Check sheet for the modelled part. Datum: model origin and axes. Units: mm. A direction names the side the tool comes from. Give positions to 0.01 mm unless a question says otherwise; leave off trailing zeros. Order: outer loops, then holes, each group sorted by start corner. A loop starts at its lowest first (then second) coordinate and runs counter-clockwise, first axis right, second up. Notation, with made-up numbers: M 40,34 L 61,34 A25 ccw 61,57 Z; hole C 13,-3.75 d9. An arc over 180 degrees is marked long. Return JSON: item names as keys, results as strings. Group by question number.
from build123d import *

# Parameters (mm, degrees)
SKETCH5_W                     = 15.875
SKETCH5_H                     = 79.375
SKETCH7_W                     = 3.4
SKETCH7_H                     = 69.85
DRIVE_PIN_HOLES_PATTERN_COUNT = 4
FLANGE_SUPPORT_CUT_REACH      = 104.834
SKETCH8_R                     = 52.5
BRAKE_HAT_HEX_DEPTH           = 4.7625
F_5_16_CLEARNCE_D             = 8.2042
SKETCH11_R                    = 3.175
TRIPOD_PINS_DEPTH             = 12.7
FILLET1_R                     = 3.175
CIRPATTERN1_COUNT             = 4
SKETCH28_R                    = 48.1625
BOSS_EXTRUDE1_DEPTH           = 11.43
SKETCH29_R                    = 47.625
BOSS_EXTRUDE2_DEPTH           = 4.7625


with BuildPart() as part:
    # Sketch1 → Bearing Shaft/Flange Support (revolve)
    with BuildSketch(Plane(origin=(0, 0, 0), x_dir=(0, 0, -1), z_dir=(1, 0, 0)), mode=Mode.PRIVATE) as bearing_shaft_flange_support_sk:
        Polygon((0, 0), (-25.0825, 0), (-25.0825, -12.319), (-47.625, -12.319), (-47.625, -17.0815), (-25.0825, -17.0815), (-15.875, -17.0815), (-15.875, -70.64248), (-15.367, -71.15048), (0, -71.15048), align=None)
    revolve(bearing_shaft_flange_support_sk.sketch.rotate(Axis((0, 0, 0), (0, 1, 0)), 180), axis=Axis((0, 0, 0), (0, 1, 0)))

    # Sketch2 → Drive Pin Support (revolve)
    with BuildSketch(Plane(origin=(0, 0, 0), x_dir=(0, 0, -1), z_dir=(1, 0, 0)), mode=Mode.PRIVATE) as drive_pin_support_sk:
        Polygon((0, 0), (-52.5, 0), (-52.5, 11.43), (-27.4096, 11.43), (-27.4096, 18.43), (-22.225, 18.43), (-22.225, 27.305), (-23.61946, 27.305), (-23.61946, 68.2625), (-22.03196, 69.85), (0, 69.85), align=None)
    revolve(drive_pin_support_sk.sketch.rotate(Axis((0, 0, 0), (0, 1, 0)), 180), axis=Axis((0, 0, 0), (0, 1, 0)))

    # Sketch5 → Center Mass Removal (revolve, cut)
    with BuildSketch(Plane(origin=(0, 0, 0), x_dir=(0, 0, -1), z_dir=(1, 0, 0)), mode=Mode.PRIVATE) as center_mass_removal_sk:
        with Locations((7.9375, 30.1625)):
            Rectangle(SKETCH5_W, SKETCH5_H)
    revolve(center_mass_removal_sk.sketch.rotate(Axis((0, 0, 0), (0, -1, 0)), 180), axis=Axis((0, 0, 0), (0, -1, 0)), mode=Mode.SUBTRACT)

    # Sketch7 → Drive Pin Holes (revolve, cut)
    with BuildSketch(Plane(origin=(0, 0, 40), x_dir=(0, 0, -1), z_dir=(1, 0, 0))):
        with Locations((1.7, 34.925)):
            Rectangle(SKETCH7_W, SKETCH7_H)
    drive_pin_holes = revolve(axis=Axis((0, -6.35, 40), (0, 1, 0)), mode=Mode.SUBTRACT)

    # Drive Pin Holes Pattern: Drive Pin Holes ×4 about axis
    drive_pin_holes_pattern_axis = Axis((0, 0, 0), (0, 1, 0))
    for i in range(1, DRIVE_PIN_HOLES_PATTERN_COUNT):
        add(drive_pin_holes.rotate(drive_pin_holes_pattern_axis, i * 360 / DRIVE_PIN_HOLES_PATTERN_COUNT), mode=Mode.SUBTRACT)

    # Sketch8 → Flange Support Cut (cut, up to next)
    with BuildSketch(Plane.XZ, mode=Mode.PRIVATE) as flange_support_cut_sk1:
        Circle(SKETCH8_R)
        with BuildLine():
            ThreePointArc((6.851776468, 44.436165629), (0, 48.1625), (-6.851776468, 44.436165629))
            ThreePointArc((-6.851776468, 44.436165629), (-9.964767607, 39.850591878), (-13.274865482, 35.405206349))
            ThreePointArc((-13.274865482, 35.405206349), (-33.675960454, 33.675960454), (-35.405206349, 13.274865482))
            ThreePointArc((-35.405206349, 13.274865482), (-39.850591878, 9.964767607), (-44.436165629, 6.851776468))
            ThreePointArc((-44.436165629, 6.851776468), (-48.1625, 0), (-44.436165629, -6.851776468))
            ThreePointArc((-44.436165629, -6.851776468), (-39.850591878, -9.964767607), (-35.405206349, -13.274865482))
            ThreePointArc((-35.405206349, -13.274865482), (-33.675960454, -33.675960454), (-13.274865482, -35.405206349))
            ThreePointArc((-13.274865482, -35.405206349), (-9.964767607, -39.850591878), (-6.851776468, -44.436165629))
            ThreePointArc((-6.851776468, -44.436165629), (0, -48.1625), (6.851776468, -44.436165629))
            ThreePointArc((6.851776468, -44.436165629), (9.964767607, -39.850591878), (13.274865482, -35.405206349))
            ThreePointArc((13.274865482, -35.405206349), (33.675960454, -33.675960454), (35.405206349, -13.274865482))
            ThreePointArc((35.405206349, -13.274865482), (39.850591878, -9.964767607), (44.436165629, -6.851776468))
            ThreePointArc((44.436165629, -6.851776468), (48.1625, 0), (44.436165629, 6.851776468))
            ThreePointArc((44.436165629, 6.851776468), (39.850591878, 9.964767607), (35.405206349, 13.274865482))
            ThreePointArc((35.405206349, 13.274865482), (33.675960454, 33.675960454), (13.274865482, 35.405206349))
            ThreePointArc((13.274865482, 35.405206349), (9.964767607, 39.850591878), (6.851776468, 44.436165629))
        make_face(mode=Mode.SUBTRACT)
    flange_support_cut_tool1 = extrude(flange_support_cut_sk1.sketch, amount=-FLANGE_SUPPORT_CUT_REACH, mode=Mode.PRIVATE) & part.part
    add(flange_support_cut_tool1.solids().sort_by_distance((-51.015076, 0, 0))[0], mode=Mode.SUBTRACT)

    # Sketch10 → Brake Hat Hex (cut)
    with BuildSketch(Plane.XZ.offset(17.0815)):
        with BuildLine():
            ThreePointArc((5.969, -46.0375), (0.002019456, -40.068500342), (-5.968998634, -46.033461088))
            Line((-5.968998634, -46.033461088), (-12.209057508, -46.033461088))
            ThreePointArc((-12.209057508, -46.033461088), (-0.007882397, -47.624999348), (12.193818875, -46.0375))
            Line((12.193818875, -46.0375), (5.969, -46.0375))
        make_face()
        with BuildLine():
            ThreePointArc((-33.772735089, -33.578906915), (-23.81932603, -41.240518092), (-12.209057508, -46.033461088))
            ThreePointArc((-12.209057508, -46.033461088), (-17.890731283, -30.975814606), (-33.772735089, -33.578906915))
        make_face()
        with BuildLine():
            ThreePointArc((-45.970675481, -12.443376586), (-41.248400489, -23.805673317), (-33.772735089, -33.578906915))
            Line((-33.772735089, -33.578906915), (-36.885144527, -28.188055635))
            ThreePointArc((-36.885144527, -28.188055635), (-34.699329459, -20.035999071), (-42.850646043, -17.847426092))
            Line((-42.850646043, -17.847426092), (-45.970675481, -12.443376586))
        make_face()
        with BuildLine():
            ThreePointArc((33.761617972, -33.590084503), (17.88047671, -30.981735086), (12.193818875, -46.0375))
            ThreePointArc((12.193818875, -46.0375), (23.805673317, -41.248400489), (33.761617972, -33.590084503))
        make_face()
        with BuildLine():
            ThreePointArc((-45.966553964, 12.458593085), (-47.624999348, 0.007882397), (-45.970675481, -12.443376586))
            ThreePointArc((-45.970675481, -12.443376586), (-35.771207993, 0.005920481), (-45.966553964, 12.458593085))
        make_face()
        with BuildLine():
            Line((36.88164741, -28.186034996), (33.761617972, -33.590084503))
            ThreePointArc((33.761617972, -33.590084503), (41.240518092, -23.81932603), (45.966553964, -12.458593085))
            Line((45.966553964, -12.458593085), (42.854144527, -17.849444365))
            ThreePointArc((42.854144527, -17.849444365), (34.701348915, -20.032501271), (36.88164741, -28.186034996))
        make_face()
        with BuildLine():
            ThreePointArc((-33.761617972, 33.590084503), (-41.240518092, 23.81932603), (-45.966553964, 12.458593085))
            Line((-45.966553964, 12.458593085), (-42.854144527, 17.849444365))
            ThreePointArc((-42.854144527, 17.849444365), (-34.701348915, 20.032501271), (-36.88164741, 28.186034996))
            Line((-36.88164741, 28.186034996), (-33.761617972, 33.590084503))
        make_face()
        with BuildLine():
            ThreePointArc((45.970675481, 12.443376586), (35.771207993, -0.005920481), (45.966553964, -12.458593085))
            ThreePointArc((45.966553964, -12.458593085), (47.624999348, -0.007882397), (45.970675481, 12.443376586))
        make_face()
        with BuildLine():
            ThreePointArc((-12.193818875, 46.0375), (-23.805673317, 41.248400489), (-33.761617972, 33.590084503))
            ThreePointArc((-33.761617972, 33.590084503), (-17.88047671, 30.981735086), (-12.193818875, 46.0375))
        make_face()
        with BuildLine():
            Line((42.850646043, 17.847426092), (45.970675481, 12.443376586))
            ThreePointArc((45.970675481, 12.443376586), (41.248400489, 23.805673317), (33.772735089, 33.578906915))
            Line((33.772735089, 33.578906915), (36.885144527, 28.188055635))
            ThreePointArc((36.885144527, 28.188055635), (34.699329459, 20.035999071), (42.850646043, 17.847426092))
        make_face()
        with BuildLine():
            ThreePointArc((12.209057508, 46.033461088), (0.007882397, 47.624999348), (-12.193818875, 46.0375))
            Line((-12.193818875, 46.0375), (-5.969, 46.0375))
            ThreePointArc((-5.969, 46.0375), (-0.002019456, 40.068500342), (5.968998634, 46.033461088))
            Line((5.968998634, 46.033461088), (12.209057508, 46.033461088))
        make_face()
        with BuildLine():
            ThreePointArc((12.209057508, 46.033461088), (17.890731283, 30.975814606), (33.772735089, 33.578906915))
            ThreePointArc((33.772735089, 33.578906915), (23.81932603, 41.240518092), (12.209057508, 46.033461088))
        make_face()
    extrude(amount=-BRAKE_HAT_HEX_DEPTH, mode=Mode.SUBTRACT)

    # 5/16 Clearnce (through all)
    with Locations(Plane(origin=(0, -71.15048, 0), x_dir=(-1, 0, 0), z_dir=(0, -1, 0))):
        with Locations((0, 0)):
            Hole(F_5_16_CLEARNCE_D / 2)

    # Sketch11 → Tripod Pins (cut)
    with BuildSketch(Plane.XZ.offset(71.15048)):
        with Locations(Location((0, 9.525, 0), (0, 0, 270))):
            Circle(SKETCH11_R)
    tripod_pins = extrude(amount=-TRIPOD_PINS_DEPTH, mode=Mode.SUBTRACT)

    # Fillet1
    fillet1_edges = [part.edges().sort_by_distance(p)[0] for p in [
        (-35.405206349, 5.715, -13.274865482),
        (-13.274865482, 5.715, -35.405206349),
        (13.274865482, 5.715, -35.405206349),
        (35.405206349, 5.715, -13.274865482),
        (35.405206349, 5.715, 13.274865482),
        (13.274865482, 5.715, 35.405206349),
        (-13.274865482, 5.715, 35.405206349),
        (-35.405206349, 5.715, 13.274865482),
    ]]
    fillet(fillet1_edges, radius=FILLET1_R)

    # CirPattern1: Tripod Pins ×4 about axis
    cirpattern1_axis = Axis((0, 0, 0), (0, 1, 0))
    for i in range(1, CIRPATTERN1_COUNT):
        add(tripod_pins.rotate(cirpattern1_axis, i * 360 / CIRPATTERN1_COUNT), mode=Mode.SUBTRACT)

    # Sketch28 → Boss-Extrude1 (add)
    with BuildSketch(Plane(origin=(0, 11.43, 0), x_dir=(1, 0, 0), z_dir=(0, 1, 0))):
        with Locations(Location((0, 0, 0), (0, 0, 270))):
            Circle(SKETCH28_R)
    extrude(amount=-BOSS_EXTRUDE1_DEPTH)

    # Sketch29 → Boss-Extrude2 (add)
    with BuildSketch(Plane(origin=(0, -12.319, 0), x_dir=(1, 0, 0), z_dir=(0, 1, 0))):
        with Locations(Location((0, 0, 0), (0, 0, 270))):
            Circle(SKETCH29_R)
    extrude(amount=-BOSS_EXTRUDE2_DEPTH)


solid = part.part
1) Tool access check on faces 4 (the face through (0, 0, 0)), 5 (the face through (-0.1, -64.9, -12.7)), 6 (the face through (24.317, 14.979, -12.648)), 7 (the face through (15, 69.85, -6)). Record the directions out of +Z, -Z, +X, -X, +Y, -Y that give a thin tool (end or side, any length) a straight path to the whole face; none if there is none.
2) Release check for a two-part mould opening along Y. For faces 1 (the face through (-46.492, -14.667, -10.324)), 2 (the face through (-10, -58.45, 0)), 3 (the face through (-0.889, -10.902, 4.005)) record: released by +Y, released by -Y, zero draft, split by the parting line, or undercut.
3) Sectioned sample at D-D on y = 57. Record the boundary of the cut face in (x, z) (3 decimals), then the cut area to 3 significant figures.
4) Depth check by flat-ended pin: P1, Ø12, axis at y = 5, z = -21.5, coming from the -X side; P2, Ø5, axis at x = 0, z = 9.525, coming from the -Y side; P3, Ø1.5, axis at x = 11.5, z = -3.5, coming from the +Y side. Enter the tip coordinate at first touch or a pass-through.
5) Sectioned sample at A-A on x = 42.5. Record the boundary of the cut face in (y, z), then the cut area to 3 significant figures.
6) Material ranges on line 1 along Y through (x, z) = (34, -21); line 2 along Y through (x, z) = (13, 1) (3 decimals); line 3 along Z through (x, y) = (-0.5, 53.5), recorded low to high.
7) Sectioned sample at C-C on z = -30.5. Record the boundary of the cut face in (x, y), then the cut area to 3 significant figures.
8) Sectioned sample at B-B on y = -61.5. Record the boundary of the cut face in (x, z) (3 decimals), then the cut area to 3 significant figures.
Reply:
{
 "1": {"face 4": "none", "face 5": "-Y", "face 6": "+Y", "face 7": "+Z, -Z, +X, -X, +Y"},
 "2": {"face 1": "zero draft", "face 2": "released by -Y", "face 3": "undercut"},
 "3": {"outline": "C 0,0 d47.239; hole C 0,0 d31.75", "area": "961 mm^2"},
 "4": {"P1": "x = -45.6", "P2": "y = -58.45", "P3": "y = 11.43"},
 "5": {"outline": "M -17.08,-21.49 L -12.32,-21.49 L -12.32,21.49 L -17.08,21.49 Z; M 0,-22.66 L 11.43,-22.66 L 11.43,22.66 L 0,22.66 Z", "area": "723 mm^2"},
 "6": {"line 1": "-17.08 to -12.32, 0 to 11.43", "line 2": "-71.15 to -9.525, 0 to 11.43", "line 3": "-23.61 to -15.87, 15.87 to 23.61"},
 "7": {"outline": "M -37.27,0 L 37.27,0 L 37.27,11.43 L -37.27,11.43 Z; M -36.58,-17.08 L 36.58,-17.08 L 36.58,-12.32 L -36.58,-12.32 Z", "area": "1,200 mm^2"},
 "8": {"outline": "C 0,0 d31.75; hole C -9.525,0 d6.35; hole C 0,0 d8.204; hole C 0,-9.525 d6.35; hole C 0,9.525 d6.35; hole C 9.525,0 d6.35", "area": "612 mm^2"}
}
